Geometry: final body of the model. Coordinates: model frame, mm. A direction names the side the tool comes from. Round coordinates to 2 decimals unless told otherwise and drop trailing zeros. Write each loop counter-clockwise with the first axis right and the second up, starting at its lowest first coordinate (ties: lowest second). Pieces come first, ordered by that corner, then holes. Notation, with made-up numbers: M 25,13 L 29,13 A20 ccw 29,38 Z; hole C -7.75,-7.75 d8. An arc over 180 degrees is marked long. Put each result on its own line as item: value. Start each with the question number.
```python
from build123d import *

# Parameters (mm, degrees)
SKETCH_1_R          = 6
EXTRUDE_1_DEPTH     = 3.8
SKETCH_2_R          = 4
EXTRUDE_2_DEPTH     = 10
SKETCH_3_R          = 3
EXTRUDE_3_DEPTH     = 8
SKETCH_4_W          = 1.8
SKETCH_4_H          = 13.920962764
CUT_EXTRUDE_1_DEPTH = 1.8


with BuildPart() as part:
    # 草图1 → 凸台-拉伸1 (new body)
    with BuildSketch(Plane(origin=(0, 0, 0), x_dir=(1, 0, 0), z_dir=(0, 1, 0))):
        with Locations(Location((0, 0, 0), (0, 0, 90))):
            Circle(SKETCH_1_R)
    extrude(amount=EXTRUDE_1_DEPTH)

    # 草图2 → 凸台-拉伸2 (add)
    with BuildSketch(Plane(origin=(0, 3.8, 0), x_dir=(1, 0, 0), z_dir=(0, 1, 0))):
        with Locations(Location((0, 0, 0), (0, 0, 270))):
            Circle(SKETCH_2_R)
    extrude(amount=EXTRUDE_2_DEPTH)

    # 草图3 → 凸台-拉伸3 (add)
    with BuildSketch(Plane(origin=(0, 13.8, 0), x_dir=(1, 0, 0), z_dir=(0, 1, 0))):
        with Locations(Location((0, 0, 0), (0, 0, 270))):
            Circle(SKETCH_3_R)
    extrude(amount=EXTRUDE_3_DEPTH)

    # 草图4 → 切除-拉伸1 (cut)
    with BuildSketch(Plane.XZ):
        Rectangle(SKETCH_4_W, SKETCH_4_H)
    extrude(amount=-CUT_EXTRUDE_1_DEPTH, mode=Mode.SUBTRACT)


solid = part.part
```
1) First-contact query: pin 1 (3 mm diameter, centred on x = 4, y = 18, fed in from +Z); pin 2 (2 mm diameter, centred on x = -3, y = 9.5, fed in from +Z); pin 3 (4 mm diameter, centred on x = -4.5, y = 11, fed in from -Z). Flat tips, straight axial feed; report the tip coordinate or a pass-through.
2) Section B-B, the plane z = 0. Output: boundary loops of the cut face in (x, y).
3) Access query for faces 1 (the face through (0, 1.8, 0)), 2 (the face through (3.92, 3.8, 1.42)), 3 (the face through (3, 0, 0)). Directions: +Z, -Z, +X, -X, +Y, -Y. A direction counts if a zero-diameter tool reaches every point of the face in a straight line with its end or side. Return the directions, or none.
4) Section D-D, the plane z = -4.75. Output: boundary loops of the cut face in (x, y), and give its area (3 significant figures).
5) Section C-C, the plane y = 18. Output: boundary loops of the cut face in (x, z), and give its area (3 significant figures).
6) Section A-A, the plane x = 0. Output: boundary loops of the cut face in (y, z).
7) Draft query along X for faces 4 (the face through (-1.802, 1.873, -5.723)), 5 (the face through (0.9, 1, 0)), 6 (the face through (-3, 0, 0)). Return one class per face: +X half, -X half, draft (parallel to the pull), parting line (faces both ways), or undercut.
8) Ray query, probe 1 along Y at (x, z) = (-0.5, -2.5); probe 2 along Y at (x, z) = (-3.75, -1.5); probe 3 along X at (y, z) = (7, 0). Return the intervals inside material, ascending.
Solved:
1. pin 1: stops at z = 1.66
1. pin 2: stops at z = 3.46
1. pin 3: stops at z = -3.12
2. outline: M -6,0 L -0.9,0 L -0.9,1.8 L 0.9,1.8 L 0.9,0 L 6,0 L 6,3.8 L 4,3.8 L 4,13.8 L 3,13.8 L 3,21.8 L -3,21.8 L -3,13.8 L -4,13.8 L -4,3.8 L -6,3.8 Z
3. face 1: +Z, -Z, -Y
3. face 2: +Y
3. face 3: +Z, -Z, +X, -X, -Y
4. outline: M -3.67,0 L -0.9,0 L -0.9,1.8 L 0.9,1.8 L 0.9,0 L 3.67,0 L 3.67,3.8 L -3.67,3.8 Z
4. area: 24.6 mm2
5. outline: C 0,0 d6
5. area: 28.3 mm2
6. outline: M 1.8,-6 L 3.8,-6 L 3.8,-4 L 13.8,-4 L 13.8,-3 L 21.8,-3 L 21.8,3 L 13.8,3 L 13.8,4 L 3.8,4 L 3.8,6 L 1.8,6 Z
7. face 4: parting line
7. face 5: undercut
7. face 6: draft
8. probe 1: y = 1.8 to 21.8
8. probe 2: y = 0 to 3.8
8. probe 3: x = -4 to 4
